Part model, mm, in its own coordinate system. Face numbers are marked on the shaded views. A direction names the side the tool comes from. Round coordinates to 2 decimals unless told otherwise and drop trailing zeros. Write each loop counter-clockwise with the first axis right and the second up, starting at its lowest first coordinate (ties: lowest second). Pieces come first, ordered by that corner, then holes. Notation, with made-up numbers: M -29,8.5 L 21,8.5 A20 ccw 21,24.5 Z; hole C 45.5,11 d5. An arc over 180 degrees is marked long. Use one line per item in the form item = value. Start each with the question number.
Item 1: Mould opens along Z. For the marked faces 4, 5 and 6 say: +Z half, -Z half, draft (parallel to the pull), parting line (faces both ways), or undercut.
Item 2: Cut at D-D, the plane z = -112.5. Give the cut face in (x, y).
Item 3: Which spindle directions (+Z, -Z, +X, -X, +Y, -Y) get a long thin tool onto all of the face, cutting with end or side? Do the marked faces 1, 2 and 3. Say none if no direction does.
Item 4: Flat gauge pins, fed straight in: pin 1 Ø6 at (x, y) = (-36, 8) entering from +Z; pin 2 Ø0.6 at (y, z) = (0, -109.5) entering from +X; pin 3 Ø2 at (y, z) = (4, -108) entering from -X. Where does each tip first touch, or does it go through?
Item 5: Cut at C-C, the plane y = 15. Give the cut face in (x, z).
Item 6: Probe L1, parallel to Y at x = -30, z = -105; L2, parallel to Y at x = -33, z = -109.5; L3, parallel to Z at x = -35, y = 18.25. List the from-to ranges inside material, lowest first.
Item 7: Cut at A-A, the plane z = -103.5. Give the cut face in (x, y).
Item 8: Cut at B-B, the plane x = -39. Give the cut face in (y, z), then the cut area to 3 significant figures.
from build123d import *

# Parameters (mm, degrees)
SALIENTE_EXTRUIR1_DEPTH = 1.5
SKETCH1_R               = 2.2
BOSS_EXTRUDE1_DEPTH     = 21.500000004
FILLET1_R               = 1
BOSS_EXTRUDE2_DEPTH     = 0.5
SKETCH3_W               = 5
SKETCH3_H               = 5
CUT_EXTRUDE1_DEPTH      = 0.5


with BuildPart() as part:
    # Croquis1 → Saliente-Extruir1 (new body)
    with BuildSketch(Plane(origin=(0, 0, 0), x_dir=(1, 0, 0), z_dir=(0, 1, 0))):
        with BuildLine():
            Line((-28.127006156, 104.147953484), (-32.167734628, 102.755086599))
            ThreePointArc((-32.167734628, 102.755086599), (-38.119150085, 113.660211034), (-28.911320585, 105.320129452))
            ThreePointArc((-28.911320585, 105.320129452), (-28.527159067, 104.728691469), (-28.127006156, 104.147953484))
        make_face()
    extrude(amount=SALIENTE_EXTRUIR1_DEPTH)

    # Sketch1 → Boss-Extrude1 (add)
    with BuildSketch(Plane(origin=(0, 1.5, 0), x_dir=(1, 0, 0), z_dir=(0, 1, 0))):
        with Locations(Location((-34.220833362, 108.71115792, 0), (0, 0, 270))):
            Circle(SKETCH1_R)
    extrude(amount=BOSS_EXTRUDE1_DEPTH)

    # Fillet1
    fillet1_edges = [part.edges().sort_by_distance(p)[0] for p in [
        (-34.220833362, 1.5, -110.91115792),
    ]]
    fillet(fillet1_edges, radius=FILLET1_R)

    # Sketch2 → Boss-Extrude2 (add)
    with BuildSketch(Plane(origin=(0, 1.5, 0), x_dir=(1, 0, 0), z_dir=(0, 1, 0))):
        with BuildLine():
            Line((-28.127006156, 104.147953484), (-32.167734628, 102.755086599))
            ThreePointArc((-32.167734628, 102.755086599), (-40.517997562, 108.522152547), (-32.528643989, 114.779641679))
            Line((-32.528643989, 114.779641679), (-32.343112299, 113.800939457))
            ThreePointArc((-32.343112299, 113.800939457), (-32.430302685, 113.242017247), (-32.865386144, 112.880494657))
            Line((-32.865386144, 112.880494657), (-35.36144377, 112.020086432))
            ThreePointArc((-35.36144377, 112.020086432), (-37.529761874, 107.570547512), (-33.080222954, 105.402229408))
            Line((-33.080222954, 105.402229408), (-30.284555445, 106.36591522))
            ThreePointArc((-30.284555445, 106.36591522), (-29.746563901, 106.359998905), (-29.333985462, 106.014674515))
            ThreePointArc((-29.333985462, 106.014674515), (-28.750570862, 105.068333927), (-28.127006156, 104.147953484))
        make_face()
    extrude(amount=BOSS_EXTRUDE2_DEPTH)

    # Sketch3 → Cut-Extrude1 (cut)
    with BuildSketch(Plane.XZ):
        with Locations((-34.220833362, -108.71115792)):
            Rectangle(SKETCH3_W, SKETCH3_H)
    extrude(amount=-CUT_EXTRUDE1_DEPTH, mode=Mode.SUBTRACT)


solid = part.part
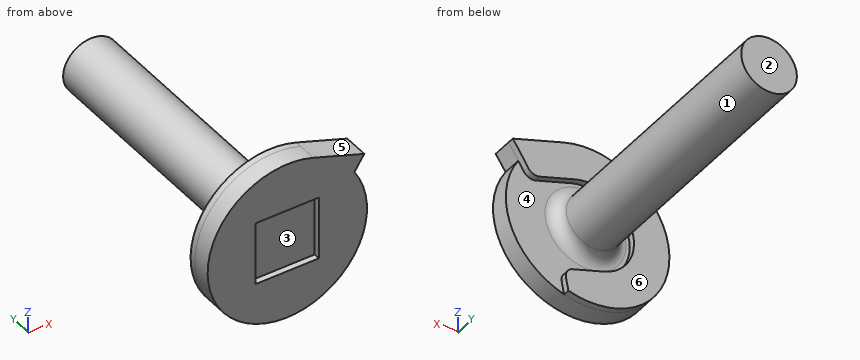
Model answer:
q1.face_4 = undercut
q1.face_5 = +Z half
q1.face_6 = draft
q2.outline = M -39.25,0 L -29.19,0 L -29.19,1.5 L -33.97,1.5 L -33.97,2 L -39.25,2 Z
q3.face_1 = +Y
q3.face_2 = +Z, -Z, +X, -X, +Y
q3.face_3 = -Y
q4.pin_1 = -106.51
q4.pin_2 = -27.94
q4.pin_3 = -36.42
q5.outline = C -34.22,-108.71 d4.4
q6.L1 = 0 to 2
q6.L2 = 0.5 to 23
q6.L3 = -110.77 to -106.65
q7.outline = M -37.76,0 L -30.01,0 L -30.01,2 L -37.76,2 Z
q8.outline = M 0,-112.82 L 2,-112.82 L 2,-104.61 L 0,-104.61 Z
q8.area = 16.4 mm²
